Check sheet for the drawn part. Datum: minimum x, y, z corner. Units: mm. A direction names the side the tool comes from. Give positions to 0.01 mm unless a question says otherwise; leave off trailing zeros. Loops run counter-clockwise (first coordinate to the right, second up) from the corner with the lowest first, then second, coordinate; pieces in that order, holes last. Notation, with made-up numbers: M 13.25,78 L 51.25,78 A26 ccw 51.25,102 Z; hole C -11.5,17 d9. An arc over 180 degrees is marked long. Write each question's results on one line, items separated by ' | '. Start each with the question number.
1. Sectioned sample at B-B on z = 19.05. Record the cut outline in (x, y) (1 decimal).
2. Material ranges on line 1 along X through (y, z) = (28.5, 6.75) (3 decimals); line 2 along X through (y, z) = (2.2, 12.7), recorded low to high.
3. Sectioned sample at D-D on y = 27. Record the cut outline in (x, z) (3 decimals), and give its area (3 significant figures).
4. Sectioned sample at C-C on x = 27. Record the cut outline in (y, z) (3 decimals), and give its area (3 significant figures).
5. Sectioned sample at A-A on z = 12.7. Record the cut outline in (x, y) (1 decimal).
6. Tool access check on the marked faces 1 and 2. Record the directions out of +Z, -Z, +X, -X, +Y, -Y that give a thin tool (end or side, any length) a straight path to the whole face; none if there is none.
7. Go/stop test with flat-tipped pins: pin 1 (4.5 mm diameter, centred on x = 28.575, z = 19.05, fed in from -Y); pin 2 (7.5 mm diameter, centred on x = 23, z = 16.5, fed in from +Y) (3 decimals); pin 3 (12 mm diameter, centred on y = 13, z = 19.5, fed in from +X) (3 decimals). Record where each tip stops, or that it passes through.
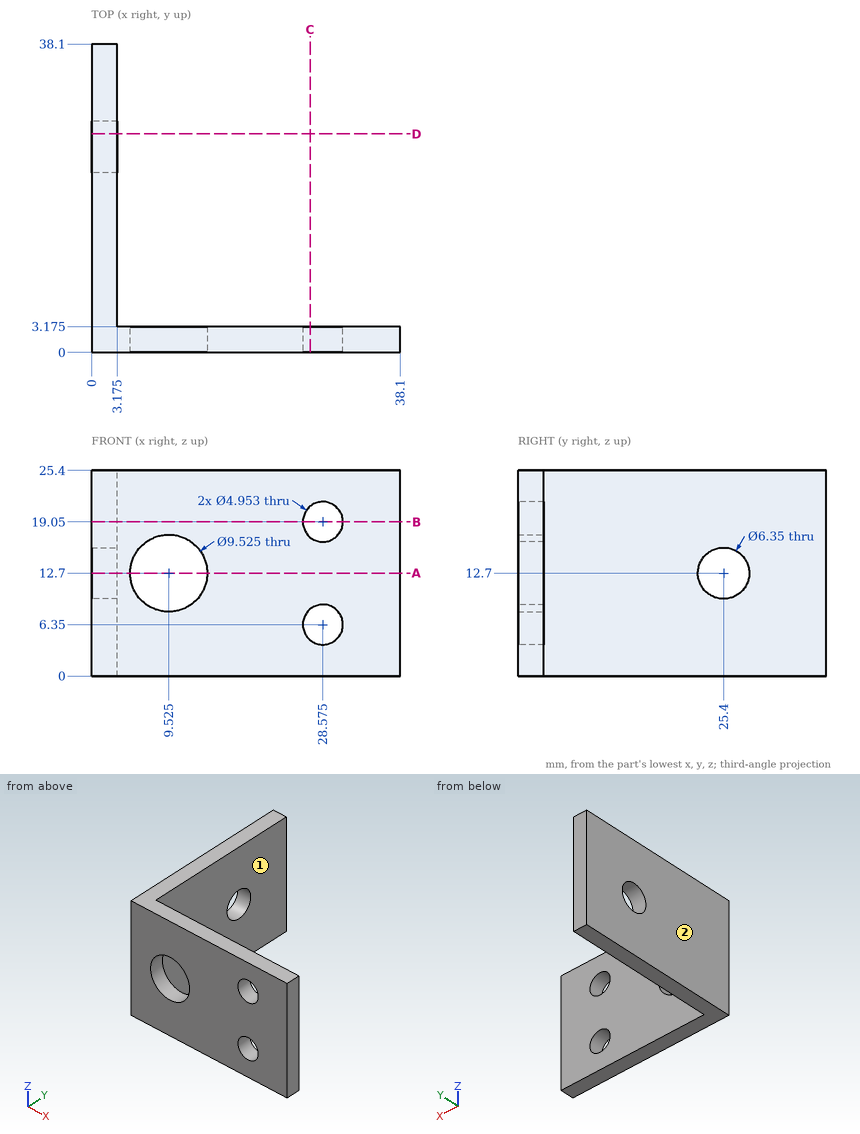
Output values:
1) outline: M 0,0 L 26.1,0 L 26.1,3.2 L 3.2,3.2 L 3.2,38.1 L 0,38.1 Z; M 31.1,0 L 38.1,0 L 38.1,3.2 L 31.1,3.2 Z
2) line 1: 0 to 3.175 | line 2: 0 to 4.76, 14.29 to 38.1
3) outline: M 0,0 L 3.175,0 L 3.175,9.958 L 0,9.958 Z; M 0,15.442 L 3.175,15.442 L 3.175,25.4 L 0,25.4 Z | area: 63.2 mm2
4) outline: M 0,0 L 3.175,0 L 3.175,4.439 L 0,4.439 Z; M 0,8.261 L 3.175,8.261 L 3.175,17.139 L 0,17.139 Z; M 0,20.961 L 3.175,20.961 L 3.175,25.4 L 0,25.4 Z | area: 56.4 mm2
5) outline: M 0,0 L 4.8,0 L 4.8,3.2 L 3.2,3.2 L 3.2,22.2 L 0,22.2 Z; M 0,28.6 L 3.2,28.6 L 3.2,38.1 L 0,38.1 Z; M 14.3,0 L 38.1,0 L 38.1,3.2 L 14.3,3.2 Z
6) face 1: +Z, -Z, +X, +Y | face 2: +Z, -Z, -X, +Y, -Y
7) pin 1: through | pin 2: y = 3.175 | pin 3: x = 3.175
